Autodesk Inventor part; units mm, degrees
ref_plane "Work Plane1" through (0, -10, 0) normal (0.8660254, 0, 0.5) x (0, 1, 0)
ref_plane "YZ Plane" through (0, 0, 0) normal (1, 0, 0) x (0, 1, 0)
ref_plane "XZ Plane" through (0, 0, 0) normal (0, 1, 0) x (-1, 0, 0)
sketch "Sketch1" plane through (0, 0, 0) normal (0, 1, 0) x (-1, 0, 0)
  circle A0 centre (0, 0) radius 1.5
  dimension "d0" = 3
extrude "Extrusion1" add sketch "Sketch1" along normal blind 78
chamfer "Chamfer1" distance 1.5 distance2 4 1 edges at (1.5, 78, 0) measured on face at (-0.3743, 78, -0.3316)
sketch "Sketch2" plane through (0, 0, 0) normal (0, -1, 0) x (1, 0, 0)
  circle A0 centre (0, 0) radius 1.5
  line L0 (2.8868, -5) -> (-2.8868, -5)
  line L1 (-2.8868, -5) -> (-5.7735, 0)
  line L2 (-5.7735, 0) -> (-2.8868, 5)
  line L3 (-2.8868, 5) -> (2.8868, 5)
  line L4 (2.8868, 5) -> (5.7735, 0)
  line L5 (5.7735, 0) -> (2.8868, -5)
  dimension "d6" = 10
extrude "Extrusion2" add sketch "Sketch2" along normal blind 11 contours A0 | L0 L1 L2 L3 L4 L5
sketch "Sketch3" plane through (0, -11, 0) normal (0, -1, 0) x (1, 0, 0)
  circle A0 centre (0, 0) radius 3
  dimension "d12" = 6
extrude "Extrusion3" add sketch "Sketch3" along normal blind 6
ref_plane "Work Plane1" through (0, -10, 0) normal (0.8660254, 0, 0.5) x (0, 1, 0)
sketch "Sketch5" plane through (0, -10, 0) normal (0.8660254, 0, 0.5) x (0, 1, 0)
  line L0 (10, 4.25) -> (5.5, 5.7735)
  line L1 (10, 5.7735) -> (10, 2.8868) construction
  line L2 (10, 5.7735) -> (-1, 5.7735) construction
  line L3 (-1, 2.8868) -> (-1, 5.7735) construction
  line L4 (10, 2.8868) -> (-1, 2.8868) construction
  line L5 (10, 4.25) -> (10, 5.7735)
  line L6 (5.5, 5.7735) -> (10, 5.7735)
  line L7 (-18.8, 0) -> (105.8, 0)
  point P0 (10, 0)
  dimension "d17" = 4.25
  dimension "d18" = 4.5
revolve "Revolution1" cut sketch "Sketch5" angle 360 about axis through (0, -10, 0) along (0, 1, 0)
sketch "Sketch7" plane through (0, 0, 0) normal (1, 0, 0) x (0, 1, 0)
  circle A0 centre (64.5, 0) radius 0.5
  line L0 (64.5, 0) -> (0, 0) construction
  dimension "d24" = 64.5
  dimension "d25" = 1
sketch "Sketch8" plane through (0, 0, 0) normal (0, 0, 1) x (1, 0, 0)
  circle A0 centre (0, 70.5) radius 0.5
  line L0 (0, 70.5) -> (0, 0) construction
  line L1 (-1.5, 0) -> (1.5, 0) construction
  dimension "d26" = 70.5
  dimension "d27" = 1
extrude "Extrusion5" cut sketch "Sketch8" along normal through all both and the other way through all
extrude "Extrusion6" cut sketch "Sketch7" along normal through all both and the other way through all
properties part number "CH_01_0003_injector"
CAD build for the part. Positions are in the model's coordinates, mm. A direction names the side the tool comes from. Round coordinates to 2 decimals unless told otherwise and drop trailing zeros. Write each loop counter-clockwise with the first axis right and the second up, starting at its lowest first coordinate (ties: lowest second). Pieces come first, ordered by that corner, then holes. Notation, with made-up numbers: (-18, 55) - (11, 55) arc R18 ccw to (11, 61) - close; hole circle Ø5 at (-36.75, -18.5). An arc over 180 degrees is marked (long way). Return JSON: item names as keys, results as strings. Group by question number.
Item 1: Band-saw the part on B-B on y = 20. List the corners of the cut face in (x, z), plus the area to 3 significant figures.
Item 2: Probe probe 1 along Z at (x, y) = (0, 34.5); probe 2 along Z at (x, y) = (-0.15, 64.5); probe 3 along Z at (x, y) = (0.95, 64.5). List the from-to ranges inside material, lowest first.
Item 3: 3-axis set-ups, long thin cutter, end or side, ignore diameter. For faces 1 (the face through (-4.35, -6.546, 2.465)), 2 (the face through (2.5, -11, 2.3)), 3 (the face through (2, 0, 0)): which of +Z, -Z, +X, -X, +Y, -Y reach the whole face in a straight line?
Item 4: Flat gauge pins, fed straight in: pin 1 Ø1.5 at (x, y) = (1, 16) entering from +Z; pin 2 Ø1 at (x, z) = (-2, 2) entering from +Y; pin 3 Ø1 at (x, z) = (-4.5, 0) entering from -Y. Where does each tip first touch, or does it go through?
Item 5: Band-saw the part on A-A on y = -10. List the corners of the cut face in (x, z), plus the area to 3 significant figures.
Resolved:
{
 "1": {"outline": "circle Ø3 at (0, 0)", "area": "7.07 mm²"},
 "2": {"probe 1": "z = -1.5 to 1.5", "probe 2": "z = -1.49 to -0.5, 0.5 to 1.49", "probe 3": "z = -1.16 to -0.5, 0.5 to 1.16"},
 "3": {"face 1": "+Z, -X, +Y, -Y", "face 2": "-Y", "face 3": "+Y"},
 "4": {"pin 1": "stops at z = 1.48", "pin 2": "stops at y = 0", "pin 3": "stops at y = -11"},
 "5": {"outline": "(-5.77, 0) - (-2.89, -5) - (2.89, -5) - (5.77, 0) - (2.89, 5) - (-2.89, 5) - close", "area": "86.6 mm²"}
}
